Autodesk Inventor part; units mm, degrees
ref_plane "YZ Plane" through (0, 0, 0) normal (1, 0, 0) x (0, 1, 0)
ref_plane "XZ Plane" through (0, 0, 0) normal (0, 1, 0) x (-1, 0, 0)
ref_plane "XY Plane" through (0, 0, 0) normal (0, 0, 1) x (1, 0, 0)
sketch "Sketch1" plane through (0, 0, 0) normal (0, 0, 1) x (1, 0, 0)
  line L0 (-11.0022, 0) -> (11.0022, 0) construction
  line L1 (0, 10.3849) -> (0, -10.3849) construction
  line L2 (0, 0) -> (0, 20)
  line L3 (0, 20) -> (3.4, 20)
  line L4 (3.4, 20) -> (3.4, 14)
  line L5 (3.4, 14) -> (5, 14)
  line L6 (5, 14) -> (5, 0)
  line L7 (5, 0) -> (0, 0)
  line L8 (0, 6) -> (5, 6)
  dimension "d0" = 40
  dimension "d1" = 28
  dimension "d2" = 1.6
  dimension "d4" = 12
  dimension "d17" = 5
revolve "Revolution1" add sketch "Sketch1" angle 360 about axis through (-11.0022, 0, 0) along (1, 0, 0) contours L2 L3 L4 L5 L6 L8
sketch "Sketch2" plane through (0, 0, 0) normal (-1, 0, 0) x (0, 0, 1)
  circle A0 centre (0, 0) radius 17 construction
  line L0 (0, 0) -> (-21.4597, 0) construction
  point P0 (-17, 0)
  dimension "d6" = 34
hole "Hole1" at (0, 0, -17) direction (1, 0, 0) diameter 2.2 depth 8 tip angle 118
pattern_circular "Circular Pattern1" count 4 over 360 about axis through (2.5, 0, 0) along (1, 0, 0) of "Hole1"
properties part number "P04" material "Aluminium"
The model under review builds one solid part; all positions refer to its coordinate system, in mm. A direction names the side the tool comes from. Give positions to 0.01 mm unless a question says otherwise; leave off trailing zeros. Order: outer loops, then holes, each group sorted by start corner. A loop starts at its lowest first (then second) coordinate and runs counter-clockwise, first axis right, second up. Notation, with made-up numbers: M -15,18.5 L -8,18.5 A19 cw -8,46.5 Z; hole C -13,-16.75 d11. An arc over 180 degrees is marked long. One line per question, with ' | ' between items. Start each with the question number.
1) Clearance check with flat-ended pins moving along their axes: P1, Ø12, axis at y = 15.5, z = -4.5, coming from the -X side; P2, Ø3, axis at y = 0, z = -17, coming from the +X side; P3, Ø1.5, axis at x = 1, z = 1.5, coming from the -Y side; P4, Ø3, axis at x = 1, y = 9.5, coming from the -Z side. State where each tip first meets the part, or that it passes through.
2) For faces 4 (the face through (4.211, 12.932, -5.362)), 5 (the face through (5, 3, -6)), list the 3-axis set-ups (+Z, -Z, +X, -X, +Y, -Y) from which the entire face can be reached by the end or side of a thin tool; tool diameter is ignored.
3) Wall thickness on L1, parallel to Y at x = 2.4, z = -1; L2, parallel to X at y = 8, z = 13; L3, parallel to Y at x = 1.85, z = 0.5: over which ranges is each line inside the solid? List them lowest first. Write a range as from..to.
4) Mouldability with a two-part tool opening along Z and no side actions: class faces 1 (the face through (0, 4, 5)), 2 (the face through (1.724, -4.336, -19.524)), 3 (the face through (1.7, 18.1, 0)) as pulls with the +Z half, pulls with the -Z half, needs draft (parallel to the pull), parting line crosses it, or undercut.
5) Consider section A-A, the plane y = 0. Give the boundary of the cut face in (x, z), then the cut area to 3 significant figures.
6) Consider section C-C, the plane y = 17. Give the boundary of the cut face in (x, z).
Found:
1) P1: stops at x = 0 | P2: stops at x = 3.4 | P3: stops at y = -19.99 | P4: stops at z = -18.33
2) face 4: +X | face 5: +Z, -Z, +X, +Y, -Y
3) L1: y = -19.97..-17.46, -16.54..-5.92, 5.92..16.54, 17.46..19.97 | L2: x = 0..3.4 | L3: y = -19.99..-17.98, -16.02..-5.98, 5.98..16.02, 17.98..19.99
4) face 1: needs draft | face 2: parting line crosses it | face 3: undercut
5) outline: M 0,-20 L 3.4,-20 L 3.4,-18.1 L 0,-18.1 Z; M 0,-15.9 L 3.4,-15.9 L 3.4,-14 L 5,-14 L 5,-6 L 0,-6 Z; M 0,6 L 5,6 L 5,14 L 3.4,14 L 3.4,15.9 L 0,15.9 Z; M 0,18.1 L 3.4,18.1 L 3.4,20 L 0,20 Z | area: 106 mm²
6) outline: M 0,-10.54 L 3.4,-10.54 L 3.4,-1.1 L 0,-1.1 Z; M 0,1.1 L 3.4,1.1 L 3.4,10.54 L 0,10.54 Z
